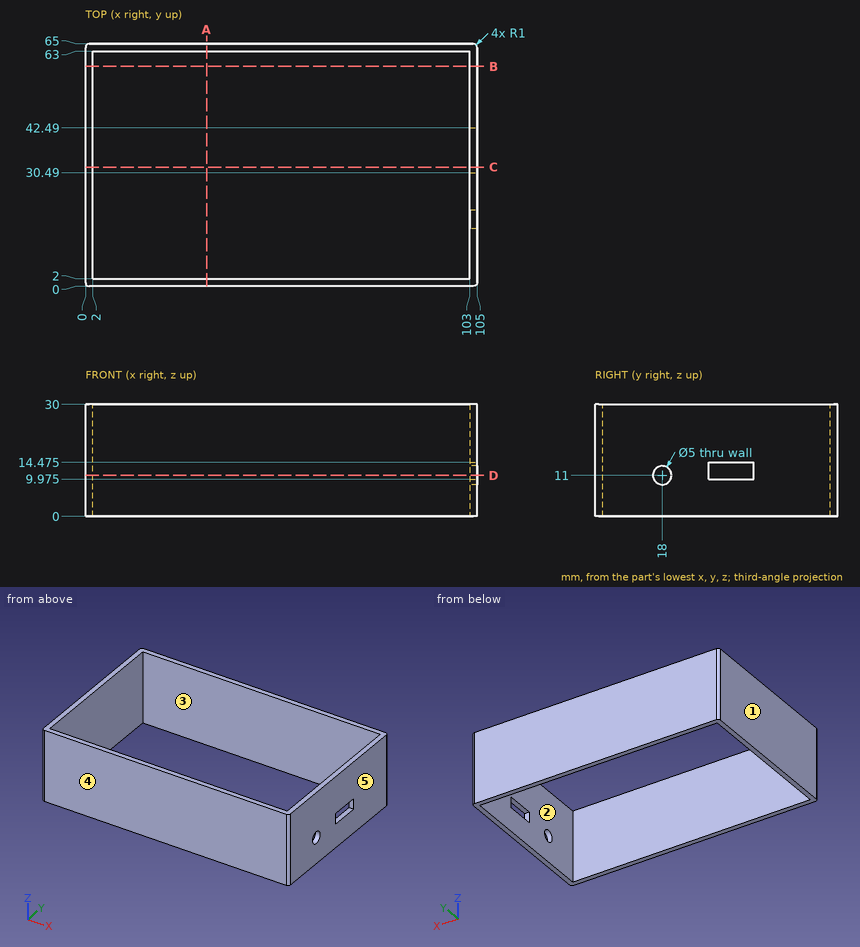
Part print with two shaded views. Sizes in mm from the minimum x, y, z corner. A direction names the side the tool comes from. Round coordinates to 2 decimals unless told otherwise and drop trailing zeros. Order: outer loops, then holes, each group sorted by start corner. A loop starts at its lowest first (then second) coordinate and runs counter-clockwise, first axis right, second up. Notation, with made-up numbers: (70, 30.25) - (116, 30.25) arc R11 ccw to (116, 34.25) - close; hole circle Ø5 at (-24.75, 75.25). An arc over 180 degrees is marked (long way). Return JSON: item names as keys, results as strings.
(1) Pin check, flat tip, straight feed: pin 1 Ø15 at (y, z) = (46.5, 9) entering from -X. Stop position of the tip, or through.
Answer key:
{"pin 1": "stops at x = 0"}
(2) Cut at A-A (x = 32.5). Give the cut face in (y, z).
Answer key:
{"outline": "(0, 0) - (2, 0) - (2, 30) - (0, 30) - close; (63, 0) - (65, 0) - (65, 30) - (63, 30) - close"}
(3) Pull direction X, two halves, no side cores. Call the marked faces 3, 4 and 5: +X half, -X half, draft (parallel to the pull), parting line (faces both ways), or undercut.
Answer key:
{"face 3": "undercut", "face 4": "draft", "face 5": "+X half"}
(4) Cut at C-C (y = 32). Give the cut face in (x, z) (1 decimal), then the cut area to 3 significant figures.
Answer key:
{"outline": "(0, 0) - (2, 0) - (2, 30) - (0, 30) - close; (103, 0) - (105, 0) - (105, 10) - (103, 10) - close; (103, 14.5) - (105, 14.5) - (105, 30) - (103, 30) - close", "area": "111 mm^2"}
(5) Cut at D-D (z = 11). Give the cut face in (x, y), then the cut area to 3 significant figures.
Answer key:
{"outline": "(0, 1) arc R1 ccw to (1, 0) - (104, 0) arc R1 ccw to (105, 1) - (105, 15.5) - (103, 15.5) - (103, 2) - (2, 2) - (2, 63) - (103, 63) - (103, 42.49) - (105, 42.49) - (105, 64) arc R1 ccw to (104, 65) - (1, 65) arc R1 ccw to (0, 64) - close; (103, 20.5) - (105, 20.5) - (105, 30.49) - (103, 30.49) - close", "area": "629 mm^2"}
(6) Tool access for the marked faces 1 and 2: list every direction of +Z, -Z, +X, -X, +Y, -Y with a clear straight run to the whole face (end or side of a thin tool).
Answer key:
{"face 1": "+Z, -Z, -X, +Y, -Y", "face 2": "+Z, -Z"}
(7) Wall check: probe 1 along X at (y, z) = (11.5, 14.25); probe 2 along Y at (x, z) = (12.5, 10.5); probe 3 along Z at (x, y) = (104, 18). Give the ranges that are in metal, low to high. Write a range as from..to.
Answer key:
{"probe 1": "x = 0..2, 103..105", "probe 2": "y = 0..2, 63..65", "probe 3": "z = 0..8.5, 13.5..30"}
(8) Cut at B-B (y = 59). Give the cut face in (x, z).
Answer key:
{"outline": "(0, 0) - (2, 0) - (2, 30) - (0, 30) - close; (103, 0) - (105, 0) - (105, 30) - (103, 30) - close"}
